Geometry: see drawing. Coordinates: mm, zero at the bounding-box minimum. Give positions to 0.01 mm unless a question says otherwise; leave off trailing zeros. Write each loop counter-clockwise with the first axis right and the second up, starting at its lowest first coordinate (ties: lowest second). Pieces come first, ordered by that corner, then holes. Notation, with made-up numbers: (4.5, 42.25) - (53.5, 42.25) arc R21 cw to (53.5, 79.25) - close; hole circle Ø10 at (-6, 57.5). An arc over 180 degrees is marked (long way). Use CSV: the item, a comma, the result in double quotes. Start each with the question number.
(1) Section B-B on y = 3.5. Output: boundary loops of the cut face in (x, z), and give its area (3 significant figures).
(2) First-contact query: pin 1 Ø2 at (x, z) = (24.5, 34) entering from +Y. Flat tip, straight axial feed; report the tip coordinate or a pass-through.
(3) Draft query along Z for the marked faces 1, 2, 3 and 4. Return one class per face: released by +Z, released by -Z, zero draft, split by the parting line, or undercut.
(4) Section A-A on z = 27.4. Output: boundary loops of the cut face in (x, y), and give its area (3 significant figures).
(5) Section D-D on x = 62.5. Output: boundary loops of the cut face in (y, z), and give its area (3 significant figures).
(6) Line query: probe 1 along X at (y, z) = (1.15, 27.4); probe 2 along Z at (x, y) = (31, 4.5); probe 3 along X at (y, z) = (2.5, 17.5). Output: solid intervals per line, ascending. Write a range as [from, to].
(7) Section C-C on x = 33.4. Output: boundary loops of the cut face in (y, z), and give its area (4 significant figures).
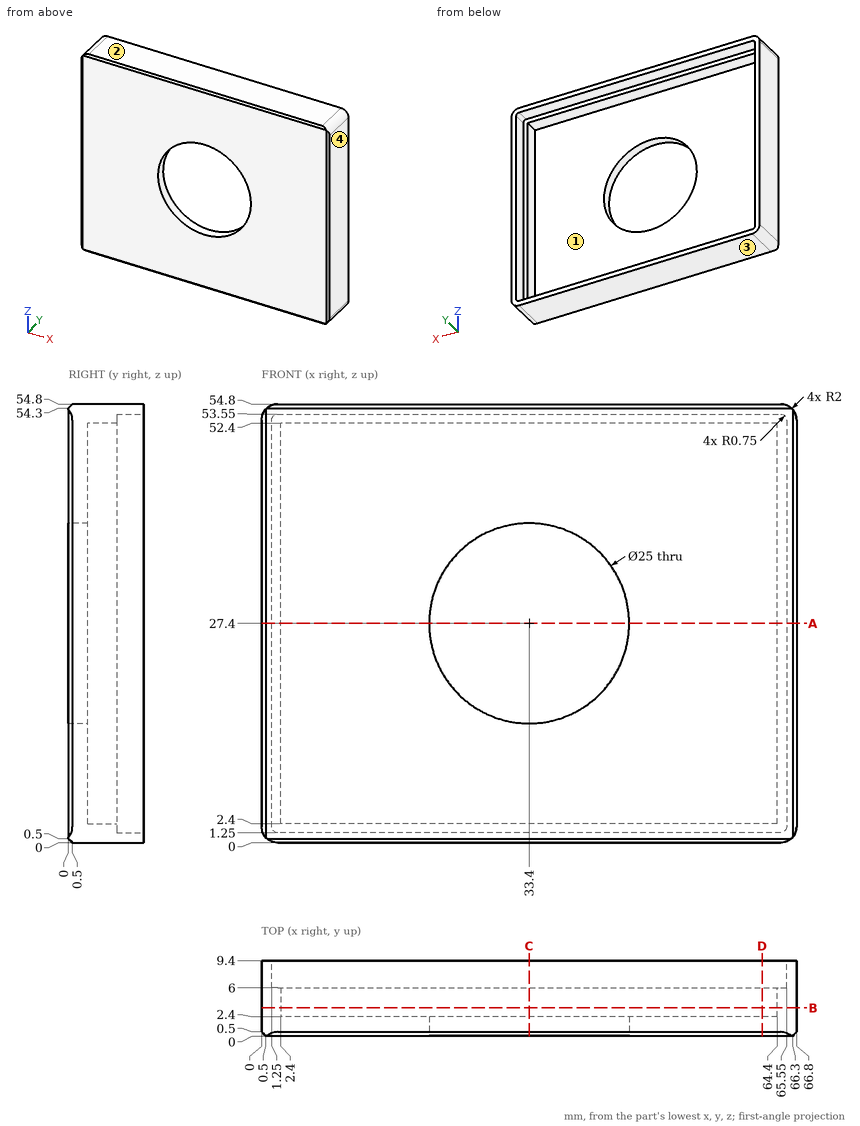
Check values:
1,outline,"(0, 2) arc R2 ccw to (2, 0) - (64.8, 0) arc R2 ccw to (66.8, 2) - (66.8, 52.8) arc R2 ccw to (64.8, 54.8) - (2, 54.8) arc R2 ccw to (0, 52.8) - close; hole (2.4, 2.4) - (64.4, 2.4) - (64.4, 52.4) - (2.4, 52.4) - close"
1,area,"557 mm²"
2,pin 1,"passes through"
3,face 1,"undercut"
3,face 2,"released by +Z"
3,face 3,"released by -Z"
3,face 4,"zero draft"
4,outline,"(0, 0.5) - (0.5, 0) - (20.9, 0) - (20.9, 2.4) - (2.4, 2.4) - (2.4, 6) - (1.25, 6) - (1.25, 9.4) - (0, 9.4) - close; (45.9, 0) - (66.3, 0) - (66.8, 0.5) - (66.8, 9.4) - (65.55, 9.4) - (65.55, 6) - (64.4, 6) - (64.4, 2.4) - (45.9, 2.4) - close"
4,area,"126 mm²"
5,outline,"(0, 0.5) - (0.5, 0) - (9.4, 0) - (9.4, 1.25) - (6, 1.25) - (6, 2.4) - (2.4, 2.4) - (2.4, 52.4) - (6, 52.4) - (6, 53.55) - (9.4, 53.55) - (9.4, 54.8) - (0.5, 54.8) - (0, 54.3) - close"
5,area,"157 mm²"
6,probe 1,"x = [0, 20.9], [45.9, 66.8]"
6,probe 2,"z = [0, 2.4], [52.4, 54.8]"
6,probe 3,"x = [0, 2.4], [64.4, 66.8]"
7,outline,"(0, 0.5) - (0.5, 0) - (9.4, 0) - (9.4, 1.25) - (6, 1.25) - (6, 2.4) - (2.4, 2.4) - (2.4, 14.9) - (0, 14.9) - close; (0, 39.9) - (2.4, 39.9) - (2.4, 52.4) - (6, 52.4) - (6, 53.55) - (9.4, 53.55) - (9.4, 54.8) - (0.5, 54.8) - (0, 54.3) - close"
7,area,"97.05 mm²"
